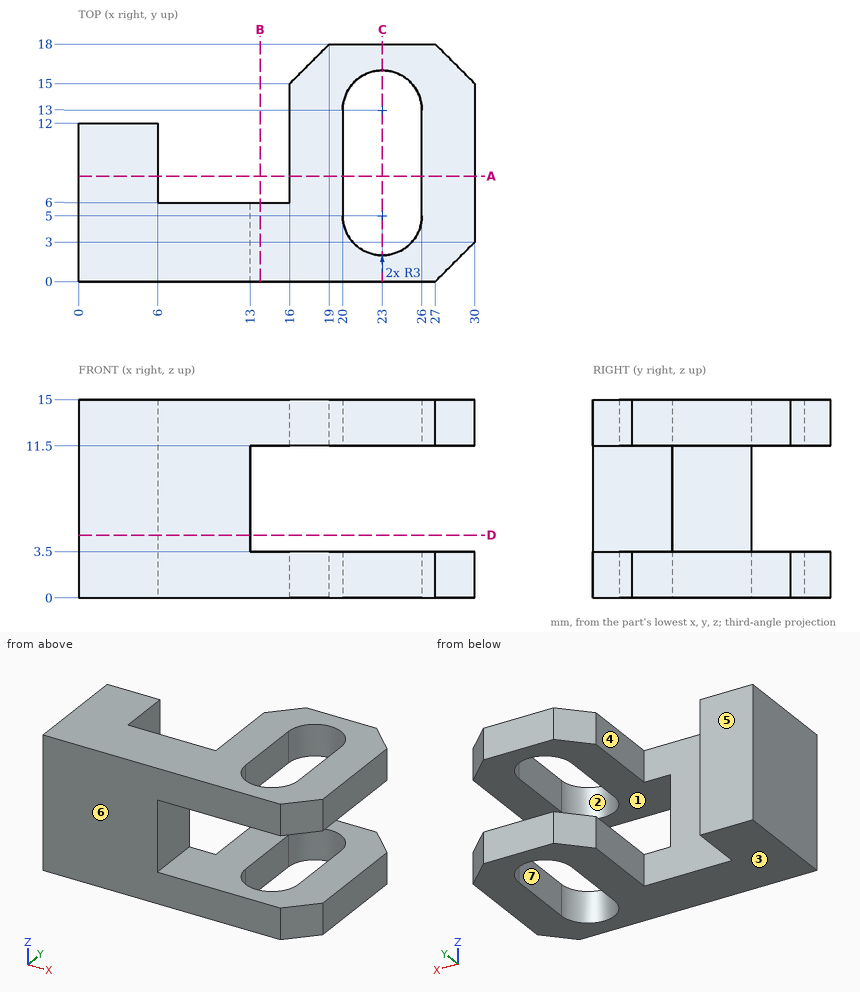
Part print with two shaded views. Sizes in mm from the minimum x, y, z corner. A direction names the side the tool comes from. Coordinates: 2 decimals unless noted, no trailing zeros. Order: outer loops, then holes, each group sorted by start corner. A loop starts at its lowest first (then second) coordinate and runs counter-clockwise, first axis right, second up. Notation, with made-up numbers: M 4,45 L 34,45 A19 cw 34,71 Z; hole C -2,-24 d9. An arc over 180 degrees is marked long. Use a Markdown table: item, result.
(1) Cut at B-B on x = 13.75. Write the cut outline in (y, z), then the cut area to 3 significant figures.
A:
| item | result |
|---|---|
| outline | M 0,0 L 6,0 L 6,3.5 L 0,3.5 Z; M 0,11.5 L 6,11.5 L 6,15 L 0,15 Z |
| area | 42.0 mm^2 |
(2) Pull direction Z, two halves, no side cores. Call the marked faces 1, 2 and 3: released by +Z, released by -Z, zero draft, split by the parting line, or undercut.
A:
| item | result |
|---|---|
| face 1 | undercut |
| face 2 | zero draft |
| face 3 | released by -Z |
(3) Cut at C-C on x = 23. Write the cut outline in (y, z), then the cut area to 3 significant figures.
A:
| item | result |
|---|---|
| outline | M 0,0 L 2,0 L 2,3.5 L 0,3.5 Z; M 0,11.5 L 2,11.5 L 2,15 L 0,15 Z; M 16,0 L 18,0 L 18,3.5 L 16,3.5 Z; M 16,11.5 L 18,11.5 L 18,15 L 16,15 Z |
| area | 28.0 mm^2 |
(4) Flat gauge pins, fed straight in: pin 1 (1.5 mm diameter, centred on y = 2.5, z = 13, fed in from -X); pin 2 (5 mm diameter, centred on x = 3, z = 4, fed in from +Y); pin 3 (1 mm diameter, centred on x = 7, z = 8.5, fed in from +Y); pin 4 (1.8 mm diameter, centred on y = 8.5, z = 10, fed in from +X). Where does each tip first touch, or does it go through?
A:
| item | result |
|---|---|
| pin 1 | stops at x = 0 |
| pin 2 | stops at y = 12 |
| pin 3 | stops at y = 6 |
| pin 4 | stops at x = 6 |
(5) Cut at D-D on z = 4.75. Write the cut outline in (x, y), then the cut area to 3 significant figures.
A:
| item | result |
|---|---|
| outline | M 0,0 L 13,0 L 13,6 L 6,6 L 6,12 L 0,12 Z |
| area | 114 mm^2 |
(6) Probe L1, parallel to X at y = 9.75, z = 14.75; L2, parallel to Z at x = 16.5, y = 12.25; L3, parallel to Y at x = 23, z = 2.25. List the from-to ranges inside material, lowest first.
A:
| item | result |
|---|---|
| L1 | x = 0 to 6, 16 to 20, 26 to 30 |
| L2 | z = 0 to 3.5, 11.5 to 15 |
| L3 | y = 0 to 2, 16 to 18 |
(7) Tool access for the marked faces 4, 5, 6 and 7: list every direction of +Z, -Z, +X, -X, +Y, -Y with a clear straight run to the whole face (end or side of a thin tool).
A:
| item | result |
|---|---|
| face 4 | +Z, -Z, +Y |
| face 5 | +Z, -Z, -X, +Y |
| face 6 | +Z, -Z, +X, -X, -Y |
| face 7 | +Z, -Z |
(8) Cut at A-A on y = 8. Write the cut outline in (x, z).
A:
| item | result |
|---|---|
| outline | M 0,0 L 6,0 L 6,15 L 0,15 Z; M 16,0 L 20,0 L 20,3.5 L 16,3.5 Z; M 16,11.5 L 20,11.5 L 20,15 L 16,15 Z; M 26,0 L 30,0 L 30,3.5 L 26,3.5 Z; M 26,11.5 L 30,11.5 L 30,15 L 26,15 Z |
